Can you work these out from the model? Positions are in its coordinate system, mm. A direction names the side the tool comes from. Round coordinates to 2 decimals unless told otherwise and drop trailing zeros. Write each loop counter-clockwise with the first axis right and the second up, starting at its lowest first coordinate (ties: lowest second). Pieces come first, ordered by that corner, then holes.
Q1. If we section it at A-A (z = 32): Please give me the cut outline in (x, y).
Q2. If we section it at D-D (x = -6.5): Please give me the cut outline in (y, z).
Q3. We'd pull the mould along X, two halves only. Please class faces 1 (the flat face through (0, 0, 0)), 2 (the flat face through (0, 0, 20)), 3 (the flat face through (30, 0, 10)): +X half, -X half, draft (parallel to the pull), parting line (faces both ways), or undercut.
Q4. Please list where these lines run through material, in increasing order: line 1 along X through (y, z) = (-3, 33); line 2 along Z through (x, y) = (23, -12); line 3 along Y through (x, z) = (-21.5, 24).
Q5. If we section it at B-B (x = 11): Please give me the cut outline in (y, z).
Q6. If we section it at C-C (y = -13): Please give me the cut outline in (x, z), plus the area to 3 significant figures.
Q7. I'm going to push flat-ended pins straight in: pin 1 Ø3.5 at (x, z) = (-25.5, 32.5) entering from +Y; pin 2 Ø24 at (y, z) = (-2.5, 33) entering from +X; pin 3 Ø12 at (x, z) = (-19, 35) entering from -Y. Where does each tip first touch, or does it pass through?
Q8. For faces 4 (the flat face through (12, -15, 35)), 5 (the flat face through (12, 15, 35)), 6 (the flat face through (18, 0, 35)), 7 (the flat face through (-18, 0, 35)), 8 (the flat face through (12, 0, 50)), which set-ups out of +Z, -Z, +X, -X, +Y, -Y let a thin tool reach every point of the face, with its end or its side?
from build123d import *

# Parameters (mm, degrees)
SKETCH_8_W      = 60
SKETCH_8_H      = 40
EXTRUDE_1_DEPTH = 20
SKETCH_9_W      = 12
SKETCH_9_H      = 30
EXTRUDE_2_DEPTH = 30
SKETCH_10_W     = 12
SKETCH_10_H     = 30
EXTRUDE_3_DEPTH = 30


with BuildPart() as part:
    # 草图8 → 凸台-拉伸1 (new body)
    with BuildSketch(Plane.XY):
        Rectangle(SKETCH_8_W, SKETCH_8_H)
    extrude(amount=EXTRUDE_1_DEPTH)

    # 草图9 → 凸台-拉伸2 (add)
    with BuildSketch(Plane.XY.offset(20)):
        with Locations((-24, 0)):
            Rectangle(SKETCH_9_W, SKETCH_9_H)
    extrude(amount=EXTRUDE_2_DEPTH)

    # 草图10 → 凸台-拉伸3 (add)
    with BuildSketch(Plane.XY.offset(20)):
        with Locations((12, 0)):
            Rectangle(SKETCH_10_W, SKETCH_10_H)
    extrude(amount=EXTRUDE_3_DEPTH)


solid = part.part
A:
1. outline: (-30, -15) - (-18, -15) - (-18, 15) - (-30, 15) - close; (6, -15) - (18, -15) - (18, 15) - (6, 15) - close
2. outline: (-20, 0) - (20, 0) - (20, 20) - (-20, 20) - close
3. face 1: draft
3. face 2: undercut
3. face 3: +X half
4. line 1: x = -30 to -18, 6 to 18
4. line 2: z = 0 to 20
4. line 3: y = -15 to 15
5. outline: (-20, 0) - (20, 0) - (20, 20) - (15, 20) - (15, 50) - (-15, 50) - (-15, 20) - (-20, 20) - close
6. outline: (-30, 0) - (30, 0) - (30, 20) - (18, 20) - (18, 50) - (6, 50) - (6, 20) - (-18, 20) - (-18, 50) - (-30, 50) - close
6. area: 1,920 mm2
7. pin 1: stops at y = 15
7. pin 2: stops at x = 18
7. pin 3: stops at y = -15
8. face 4: +Z, +X, -X, -Y
8. face 5: +Z, +X, -X, +Y
8. face 6: +Z, +X, +Y, -Y
8. face 7: +Z, +Y, -Y
8. face 8: +Z, +X, -X, +Y, -Y
